Can you work these out from the model? Positions are in its coordinate system, mm. Face numbers are marked on the shaded views. A direction names the side the tool comes from. Round coordinates to 2 decimals unless told otherwise and drop trailing zeros. Loops run counter-clockwise (first coordinate to the right, second up) from the corner with the lowest first, then second, coordinate; pieces in that order, holes last.
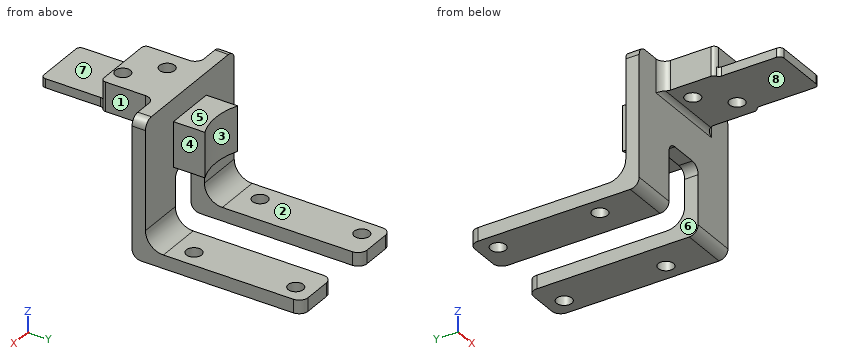
from build123d import *

# Parameters (mm, degrees)
BOSS_EXTRUDE1_DEPTH      = 3
BOSS_EXTRUDE2_DEPTH      = 35
BOSS_EXTRUDE2_DEPTH_BACK = 3
SKETCH3_W                = 10.25
SKETCH3_H                = 3
SKETCH4_W                = 15
SKETCH4_H                = 6.5
BOSS_EXTRUDE3_DEPTH      = 12
M3_CLEARANCE_HOLE1_D     = 3.4
M3_CLEARANCE_HOLE2_D     = 3.4
FILLET1_R                = 1
FILLET2_R                = 2
FILLET3_R                = 1
SKETCH11_W               = 13
SKETCH11_H               = 2
BOSS_EXTRUDE4_DEPTH      = 14
FILLET4_R                = 1
FILLET5_R                = 4
BOSS_EXTRUDE5_START      = -5
BOSS_EXTRUDE5_DEPTH      = 10


with BuildPart() as part:
    # Sketch2 → Boss-Extrude1 (new body)
    with BuildSketch(Plane(origin=(0, 0, 0), x_dir=(1, 0, 0), z_dir=(0, 1, 0))):
        Polygon((-15.25, -14), (15.25, -14), (15.25, 14), (5, 14), (5, 2), (-5, 2), (-5, 14), (-15.25, 14), align=None)
    extrude(amount=BOSS_EXTRUDE1_DEPTH)

    # Sketch3 → Boss-Extrude2 (add, two sides: drawn at the far end of the back side and taken through both)
    with BuildSketch(Plane(origin=(0, 3, 0), x_dir=(1, 0, 0), z_dir=(0, 1, 0)).offset(-BOSS_EXTRUDE2_DEPTH_BACK)):
        with Locations((-10.125, 15.5)):
            Rectangle(SKETCH3_W, SKETCH3_H)
        with Locations((10.125, 15.5)):
            Rectangle(SKETCH3_W, SKETCH3_H)
    extrude(amount=BOSS_EXTRUDE2_DEPTH + BOSS_EXTRUDE2_DEPTH_BACK)

    # Sketch4 → Boss-Extrude3 (add)
    with BuildSketch(Plane.XZ):
        with Locations((0, 10.75)):
            Rectangle(SKETCH4_W, SKETCH4_H)
    extrude(amount=BOSS_EXTRUDE3_DEPTH)

    # M3 Clearance Hole1 (through all)
    with Locations(Plane.XY.offset(14)):
        with Locations((-3, -4), (3, -10)):
            Hole(M3_CLEARANCE_HOLE1_D / 2)

    # M3 Clearance Hole2 (through all)
    with Locations(Plane.XY.offset(-14)):
        with Locations((-11.34906384, 34), (11.34906384, 34), (11.34906384, 11.30187232), (-11.34906384, 11.30187232)):
            Hole(M3_CLEARANCE_HOLE2_D / 2)

    # Fillet1
    fillet1_edges = [part.edges().sort_by_distance(p)[0] for p in [
        (-7.5, -12, 10.75),
        (7.5, -12, 10.75),
    ]]
    fillet(fillet1_edges, radius=FILLET1_R)

    # Fillet2
    fillet2_edges = [part.edges().sort_by_distance(p)[0] for p in [
        (15.25, 1.5, 14),
        (-15.25, 1.5, 14),
        (-5, 1.5, -2),
        (5, 1.5, -2),
        (-15.25, 38, -15.5),
        (-5, 38, -15.5),
        (-10.125, 0, -17),
        (15.25, 38, -15.5),
        (5, 38, -15.5),
        (10.125, 0, -17),
        (-7.5, 0, 10.75),
        (7.5, 0, 10.75),
    ]]
    fillet(fillet2_edges, radius=FILLET2_R)

    # Fillet3
    fillet3_edges = [part.edges().sort_by_distance(p)[0] for p in [
        (0, 0, 7.5),
    ]]
    fillet(fillet3_edges, radius=FILLET3_R - 0.0001)  # a hair under: the kernel refuses the full size

    # Sketch11 → Boss-Extrude4 (add)
    with BuildSketch(Plane.XZ.offset(12)):
        with Locations((0, 8.5)):
            Rectangle(SKETCH11_W, SKETCH11_H)
    extrude(amount=BOSS_EXTRUDE4_DEPTH)

    # Fillet4
    fillet4_edges = [part.edges().sort_by_distance(p)[0] for p in [
        (-6.5, -12, 8.5),
        (-6.5, -26, 8.5),
        (6.5, -26, 8.5),
        (6.5, -12, 8.5),
    ]]
    fillet(fillet4_edges, radius=FILLET4_R)

    # Fillet5
    fillet5_edges = [part.edges().sort_by_distance(p)[0] for p in [
        (-10.125, 3, -14),
        (10.125, 3, -14),
    ]]
    fillet(fillet5_edges, radius=FILLET5_R)

    # Sketch13 → Boss-Extrude5 (add)
    with BuildSketch(Plane.XY.offset(14).offset(BOSS_EXTRUDE5_START)):
        with BuildLine():
            Line((-5.637048368, 10), (-5.637048368, 3))
            Line((-5.637048368, 3), (5.637048368, 3))
            Line((5.637048368, 3), (5.637048368, 10))
            ThreePointArc((5.637048368, 10), (0, 8.800936159), (-5.637048368, 10))
        make_face()
    extrude(amount=-BOSS_EXTRUDE5_DEPTH)


solid = part.part
(1) If we section it at D-D, the plane y = -10: List the corners of the cut face in (x, z) for me, then the cut area to 3 significant figures.
Worked answers:
outline: (-7.5, 7.5) - (1.3, 7.5) - (1.3, 14) - (-7.5, 14) - close; (4.7, 7.5) - (7.5, 7.5) - (7.5, 14) - (4.7, 14) - close
area: 75.4 mm2
(2) If we mould it in two halves opening along X, with no side actions, what happens to the marked faces 1, 2 and 3? For each: released by +X, released by -X, zero draft, split by the parting line, or undercut.
Worked answers:
face 1: released by +X
face 2: zero draft
face 3: undercut
(3) Will these pins go through, and if not, where does the flat tip stop? P1, Ø8, axis at x = 11, z = -9, coming from the -Y side; P2, Ø3.5, axis at x = 1.5, y = 5, coming from the -Z side; P3, Ø8, axis at y = 13.5, z = 1.5, coming from the +X side; P4, Ø2.5, axis at x = 11.35, y = 11.3, coming from the +Z side.
Worked answers:
P1: stops at y = 0
P2: stops at z = -1
P3: stops at x = 5.64
P4: passes through
(4) If we section it at B-B, the plane y = 17: List the corners of the cut face in (x, z) for me, then the cut area to 3 significant figures.
Worked answers:
outline: (-15.25, -17) - (-5, -17) - (-5, -14) - (-15.25, -14) - close; (5, -17) - (15.25, -17) - (15.25, -14) - (5, -14) - close
area: 61.5 mm2
(5) If I drill on line 1 (Z direction, x = 8.5, y = 21); line 2 (Y direction, x = -9.5, z = 0); line 3 (Y direction, x = -0.5, z = 4), over which ranges is the centre line in solid material (lowest first)?
Worked answers:
line 1: z = -17 to -14
line 2: y = 0 to 3
line 3: y = 0 to 8.81
(6) If we section it at C-C, the plane z = 1.5: List the corners of the cut face in (x, y) for me.
Worked answers:
outline: (-15.25, 0) - (15.25, 0) - (15.25, 3) - (5.64, 3) - (5.64, 10) arc R13.85 cw to (-5.64, 10) - (-5.64, 3) - (-15.25, 3) - close
(7) If we section it at A-A, the plane y = 34: List the corners of the cut face in (x, z) for me.
Worked answers:
outline: (-15.25, -17) - (-13.05, -17) - (-13.05, -14) - (-15.25, -14) - close; (-9.65, -17) - (-5, -17) - (-5, -14) - (-9.65, -14) - close; (5, -17) - (9.65, -17) - (9.65, -14) - (5, -14) - close; (13.05, -17) - (15.25, -17) - (15.25, -14) - (13.05, -14) - close
(8) For the marked faces 4, 5, 6, 7 and 8, which set-ups out of +Z, -Z, +X, -X, +Y, -Y let a thin tool reach every point of the face, with its end or its side?
Worked answers:
face 4: +Z, +X, +Y
face 5: +Z, +X, -X, +Y
face 6: -Z, +Y, -Y
face 7: +Z, +X, -X, -Y
face 8: -Z, +X, -X, -Y
